The model under review builds one solid part; all positions refer to its coordinate system, in mm. Coordinates: 2 decimals unless noted, no trailing zeros. Write each loop counter-clockwise with the first axis right and the second up, starting at its lowest first coordinate (ties: lowest second). Pieces come first, ordered by that corner, then holes.
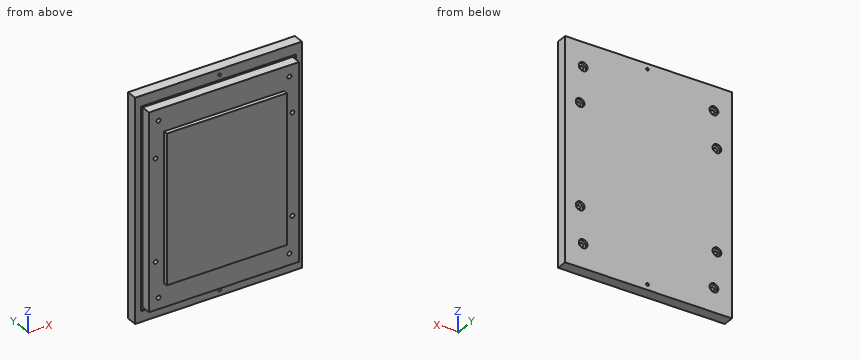
```python
from build123d import *

# Parameters (mm, degrees)
SKETCH1_W                               = 277.55
SKETCH1_H                               = 368
BOSS_EXTRUDE1_DEPTH                     = 39
SKETCH2_OUTSIDE_W                       = 372.066
SKETCH2_OUTSIDE_H                       = 462.516
SKETCH2_OUTSIDE_W_2                     = 199.55
SKETCH2_OUTSIDE_H_2                     = 247
CUT_EXTRUDE1_DEPTH                      = 7
SKETCH3_OUTSIDE_W                       = 372.066
SKETCH3_OUTSIDE_H                       = 462.516
SKETCH3_OUTSIDE_W_2                     = 249.55
SKETCH3_OUTSIDE_H_2                     = 325
CUT_EXTRUDE2_DEPTH                      = 21
CBORE_FOR_M6_HEX_HEAD_BOLT1_D           = 6.6
CBORE_FOR_M6_HEX_HEAD_BOLT1_CBORE_D     = 14.547
CBORE_FOR_M6_HEX_HEAD_BOLT1_CBORE_DEPTH = 4
SKETCH8_W                               = 257.55
SKETCH8_H                               = 333
CUT_EXTRUDE3_DEPTH                      = 2.3
SKETCH9_R                               = 2.25
CUT_EXTRUDE4_DEPTH                      = 232.420614088


with BuildPart() as part:
    # Sketch1 → Boss-Extrude1 (new body)
    with BuildSketch(Plane(origin=(0, 0, 0), x_dir=(1, 0, 0), z_dir=(0, 1, 0))):
        Rectangle(SKETCH1_W, SKETCH1_H)
    extrude(amount=BOSS_EXTRUDE1_DEPTH)

    # Sketch2 outside → Cut-Extrude1 (cut)
    with BuildSketch(Plane(origin=(0, 0, 0), x_dir=(1, 0, 0), z_dir=(0, 1, 0))):
        Rectangle(SKETCH2_OUTSIDE_W, SKETCH2_OUTSIDE_H)
        Rectangle(SKETCH2_OUTSIDE_W_2, SKETCH2_OUTSIDE_H_2, mode=Mode.SUBTRACT)
    extrude(amount=CUT_EXTRUDE1_DEPTH, mode=Mode.SUBTRACT)

    # Sketch3 outside → Cut-Extrude2 (cut)
    with BuildSketch(Plane(origin=(0, 0, 0), x_dir=(1, 0, 0), z_dir=(0, 1, 0))):
        Rectangle(SKETCH3_OUTSIDE_W, SKETCH3_OUTSIDE_H)
        Rectangle(SKETCH3_OUTSIDE_W_2, SKETCH3_OUTSIDE_H_2, mode=Mode.SUBTRACT)
    extrude(amount=CUT_EXTRUDE2_DEPTH, mode=Mode.SUBTRACT)

    # CBORE for M6 Hex Head Bolt1 (through all)
    with Locations(Plane(origin=(0, 39, 0), x_dir=(1, 0, 0), z_dir=(0, 1, 0))):
        with Locations((-108.775, -144), (-113.775, -84), (-113.775, 84), (-108.775, 144), (108.775, 144), (113.775, 84), (113.775, -84), (108.775, -144)):
            CounterBoreHole(CBORE_FOR_M6_HEX_HEAD_BOLT1_D / 2, CBORE_FOR_M6_HEX_HEAD_BOLT1_CBORE_D / 2, CBORE_FOR_M6_HEX_HEAD_BOLT1_CBORE_DEPTH)

    # Sketch8 → Cut-Extrude3 (cut)
    with BuildSketch(Plane(origin=(0, 21, 0), x_dir=(1, 0, 0), z_dir=(0, 1, 0))):
        Rectangle(SKETCH8_W, SKETCH8_H)
        with BuildLine():
            Line((124.275, 162.5), (-124.275, 162.5))
            ThreePointArc((-124.275, 162.5), (-124.628553391, 162.353553391), (-124.775, 162))
            Line((-124.775, 162), (-124.775, -162))
            ThreePointArc((-124.775, -162), (-124.628553391, -162.353553391), (-124.275, -162.5))
            Line((-124.275, -162.5), (124.275, -162.5))
            ThreePointArc((124.275, -162.5), (124.628553391, -162.353553391), (124.775, -162))
            Line((124.775, -162), (124.775, 162))
            ThreePointArc((124.775, 162), (124.628553391, 162.353553391), (124.275, 162.5))
        make_face(mode=Mode.SUBTRACT)
    extrude(amount=CUT_EXTRUDE3_DEPTH, mode=Mode.SUBTRACT)

    # Sketch9 → Cut-Extrude4 (cut, through all)
    with BuildSketch(Plane(origin=(0, 21, 0), x_dir=(-1, 0, 0), z_dir=(0, -1, 0))):
        with Locations(Location((-1.775, -175, 0), (0, 0, 90))):
            Circle(SKETCH9_R)
        with Locations(Location((-1.775, 175, 0), (0, 0, 270))):
            Circle(SKETCH9_R)
    extrude(amount=-CUT_EXTRUDE4_DEPTH, mode=Mode.SUBTRACT)


solid = part.part
```
Item 1: Take a section at A-A, the plane y = 16. Count the separate pieces of the cut face and the enclosed holes in it, plus the area to 3 significant figures.
Solved:
separate pieces: 1
enclosed holes: 8
area: 80,800 mm2
Item 2: Take a section at B-B, the plane x = 47.5. Write out the cut boundary in (y, z), plus the area to 3 significant figures.
Solved:
outline: (0, -123.5) - (7, -123.5) - (7, -162.5) - (23.3, -162.5) - (23.3, -166.5) - (21, -166.5) - (21, -184) - (39, -184) - (39, 184) - (21, 184) - (21, 166.5) - (23.3, 166.5) - (23.3, 162.5) - (7, 162.5) - (7, 123.5) - (0, 123.5) - close
area: 12,900 mm2
Item 3: Take a section at C-C, the plane z = -107. Write out the cut boundary in (x, y) (3 decimals).
Solved:
outline: (-138.775, 21) - (-128.775, 21) - (-128.775, 23.3) - (-124.775, 23.3) - (-124.775, 7) - (-99.775, 7) - (-99.775, 0) - (99.775, 0) - (99.775, 7) - (124.775, 7) - (124.775, 23.3) - (128.775, 23.3) - (128.775, 21) - (138.775, 21) - (138.775, 39) - (-138.775, 39) - close
Item 4: For pin 1 (3 mm diameter, centred on y = 19, z = 106.5, fed in from +X) (3 decimals); pin 2 (6 mm diameter, centred on x = 5, y = 8.5, fed in from -Z); pin 3 (7.5 mm diameter, centred on x = -113, z = 87, fed in from +Y), all flat-tipped, find the tip position at first contact; note any pin that passes through.
Solved:
pin 1: stops at x = 124.775
pin 2: stops at z = -162.5
pin 3: stops at y = 35
Item 5: To check wall thickness, follow line 1 along X through (y, z) = (21.5, -2) (3 decimals); line 2 along X through (y, z) = (13, -144) (3 decimals); line 3 along Z through (x, y) = (-57, 22). State the ranges of each line that lie inside material, in increasing order.
Solved:
line 1: x = -138.775 to -128.775, -124.775 to 124.775, 128.775 to 138.775
line 2: x = -124.775 to -112.075, -105.475 to 105.475, 112.075 to 124.775
line 3: z = -184 to -166.5, -162.5 to 162.5, 166.5 to 184
